from build123d import *

# Parameters (mm, degrees)
SKETCH1_W                = 59
SKETCH1_H                = 34
SKETCH1_W_2              = 55
SKETCH1_H_2              = 28
BOSS_EXTRUDE1_DEPTH      = 25
SKETCH1_2_W              = 55
SKETCH1_2_H              = 28
BOSS_EXTRUDE2_DEPTH      = 2
SKETCH2_W                = 2
SKETCH2_H                = 34
CUT_EXTRUDE1_DEPTH       = 25
SKETCH3_R                = 0.9
CUT_EXTRUDE2_DEPTH       = 25
CUT_EXTRUDE3_DEPTH       = 25
SKETCH5_W                = 2
SKETCH5_H                = 2
CUT_EXTRUDE4_DEPTH       = 51
SKETCH6_R                = 3.668845882
BOSS_EXTRUDE3_DEPTH      = 5.5
SKETCH4_3_R              = 2.4
CUT_EXTRUDE5_DEPTH       = 8
CUT_EXTRUDE5_TAPER       = -2
SKETCH7_W                = 24
SKETCH7_H                = 1.341552338
BOSS_EXTRUDE4_DEPTH      = 5.5
SKETCH8_R                = 1.5
CUT_EXTRUDE6_DEPTH       = 5.5
SKETCH9_W                = 10
SKETCH9_H                = 10
CUT_EXTRUDE7_DEPTH       = 2.5
SKETCH10_W               = 10
SKETCH10_H               = 10
CUT_EXTRUDE8_DEPTH       = 2.5
SKETCH11_R               = 1
CUT_EXTRUDE9_DEPTH       = 12.5
CUT_EXTRUDE9_DEPTH_BACK  = 2.5
SKETCH12_R               = 1
CUT_EXTRUDE10_DEPTH      = 12.5
CUT_EXTRUDE10_DEPTH_BACK = 2.5


with BuildPart() as part:
    # Sketch1 → Boss-Extrude1 (new body)
    with BuildSketch(Plane(origin=(0, 0, 0), x_dir=(1, 0, 0), z_dir=(0, 1, 0))):
        with Locations((29.5, 17)):
            Rectangle(SKETCH1_W, SKETCH1_H)
        with Locations((29.5, 17)):
            Rectangle(SKETCH1_W_2, SKETCH1_H_2, mode=Mode.SUBTRACT)
    extrude(amount=BOSS_EXTRUDE1_DEPTH)

    # Sketch1_2 → Boss-Extrude2 (add)
    with BuildSketch(Plane(origin=(0, 0, 0), x_dir=(1, 0, 0), z_dir=(0, 1, 0))):
        with Locations((29.5, 17)):
            Rectangle(SKETCH1_2_W, SKETCH1_2_H)
    extrude(amount=BOSS_EXTRUDE2_DEPTH)

    # Sketch2 → Cut-Extrude1 (cut)
    with BuildSketch(Plane(origin=(0, 25, 0), x_dir=(1, 0, 0), z_dir=(0, 1, 0))):
        with Locations((58, 17)):
            Rectangle(SKETCH2_W, SKETCH2_H)
    extrude(amount=-CUT_EXTRUDE1_DEPTH, mode=Mode.SUBTRACT)

    # Sketch3 → Cut-Extrude2 (cut)
    with BuildSketch(Plane(origin=(0, 2, 0), x_dir=(1, 0, 0), z_dir=(0, 1, 0))):
        with Locations((4, 9.5)):
            Circle(SKETCH3_R)
        with Locations((4, 24.5)):
            Circle(SKETCH3_R)
        with Locations((44.5, 9.5)):
            Circle(SKETCH3_R)
        with Locations((44.5, 24.5)):
            Circle(SKETCH3_R)
    extrude(amount=-CUT_EXTRUDE2_DEPTH, mode=Mode.SUBTRACT)

    # Sketch4 → Cut-Extrude3 (cut)
    with BuildSketch(Plane.ZY):
        with BuildLine():
            Line((-20.5, 3.8), (-13.5, 3.8))
            ThreePointArc((-13.5, 3.8), (-10.5, 6.8), (-13.5, 9.8))
            Line((-13.5, 9.8), (-20.5, 9.8))
            ThreePointArc((-20.5, 9.8), (-23.5, 6.8), (-20.5, 3.8))
        make_face()
        with BuildLine():
            Line((-24, 24.1), (-10, 24.1))
            ThreePointArc((-10, 24.1), (-9.4, 23.5), (-10, 22.9))
            Line((-10, 22.9), (-24, 22.9))
            ThreePointArc((-24, 22.9), (-24.6, 23.5), (-24, 24.1))
        make_face()
    extrude(amount=-CUT_EXTRUDE3_DEPTH, mode=Mode.SUBTRACT)

    # Sketch5 → Cut-Extrude4 (cut)
    with BuildSketch(Plane(origin=(57, 0, 0), x_dir=(0, 0, -1), z_dir=(1, 0, 0))):
        with Locations((2, 23)):
            Rectangle(SKETCH5_W, SKETCH5_H)
        with Locations((32, 23)):
            Rectangle(SKETCH5_W, SKETCH5_H)
    extrude(amount=-CUT_EXTRUDE4_DEPTH, mode=Mode.SUBTRACT)

    # Sketch6 → Boss-Extrude3 (add)
    with BuildSketch(Plane(origin=(2, 0, 0), x_dir=(0, 0, -1), z_dir=(1, 0, 0))):
        with Locations((17, 18)):
            Circle(SKETCH6_R)
    extrude(amount=BOSS_EXTRUDE3_DEPTH)

    # Sketch4_3 → Cut-Extrude5 (cut)
    with BuildSketch(Plane.ZY):
        with Locations((-17, 18)):
            Circle(SKETCH4_3_R)
        with BuildLine():
            ThreePointArc((-20.5, 9.8), (-23.5, 6.8), (-20.5, 3.8))
            Line((-20.5, 3.8), (-13.5, 3.8))
            ThreePointArc((-13.5, 3.8), (-10.5, 6.8), (-13.5, 9.8))
            Line((-13.5, 9.8), (-20.5, 9.8))
        make_face()
        with BuildLine():
            ThreePointArc((-24, 24.1), (-24.6, 23.5), (-24, 22.9))
            Line((-24, 22.9), (-10, 22.9))
            ThreePointArc((-10, 22.9), (-9.4, 23.5), (-10, 24.1))
            Line((-10, 24.1), (-24, 24.1))
        make_face()
    extrude(amount=-CUT_EXTRUDE5_DEPTH, taper=CUT_EXTRUDE5_TAPER, mode=Mode.SUBTRACT)

    # Sketch7 → Boss-Extrude4 (add)
    with BuildSketch(Plane(origin=(2, 0, 0), x_dir=(0, 0, -1), z_dir=(1, 0, 0))):
        with Locations((17, 21.329223831)):
            Rectangle(SKETCH7_W, SKETCH7_H)
    extrude(amount=BOSS_EXTRUDE4_DEPTH)

    # Sketch8 → Cut-Extrude6 (cut)
    with BuildSketch(Plane(origin=(0, 22, 0), x_dir=(1, 0, 0), z_dir=(0, 1, 0))):
        with Locations((5, 27)):
            Circle(SKETCH8_R)
        with Locations((5, 7)):
            Circle(SKETCH8_R)
    extrude(amount=-CUT_EXTRUDE6_DEPTH, mode=Mode.SUBTRACT)

    # Sketch9 → Cut-Extrude7 (cut)
    with BuildSketch(Plane(origin=(0, 0, -34), x_dir=(-1, 0, 0), z_dir=(0, 0, -1))):
        with Locations((-52, 13)):
            Rectangle(SKETCH9_W, SKETCH9_H)
    extrude(amount=-CUT_EXTRUDE7_DEPTH, mode=Mode.SUBTRACT)

    # Sketch10 → Cut-Extrude8 (cut)
    with BuildSketch(Plane.XY):
        with Locations((52, 13)):
            Rectangle(SKETCH10_W, SKETCH10_H)
    extrude(amount=-CUT_EXTRUDE8_DEPTH, mode=Mode.SUBTRACT)

    # Sketch11 → Cut-Extrude9 (cut, two sides)
    with BuildSketch(Plane(origin=(0, 18, 0), x_dir=(-1, 0, 0), z_dir=(0, -1, 0))) as cut_extrude9_sk:
        with Locations((-49, 1.3)):
            Circle(SKETCH11_R)
    extrude(amount=CUT_EXTRUDE9_DEPTH, mode=Mode.SUBTRACT)
    extrude(cut_extrude9_sk.sketch, amount=-CUT_EXTRUDE9_DEPTH_BACK, mode=Mode.SUBTRACT)

    # Sketch12 → Cut-Extrude10 (cut, two sides)
    with BuildSketch(Plane(origin=(0, 18, 0), x_dir=(-1, 0, 0), z_dir=(0, -1, 0))) as cut_extrude10_sk:
        with Locations((-48.8, 32.7)):
            Circle(SKETCH12_R)
    extrude(amount=CUT_EXTRUDE10_DEPTH, mode=Mode.SUBTRACT)
    extrude(cut_extrude10_sk.sketch, amount=-CUT_EXTRUDE10_DEPTH_BACK, mode=Mode.SUBTRACT)


solid = part.part
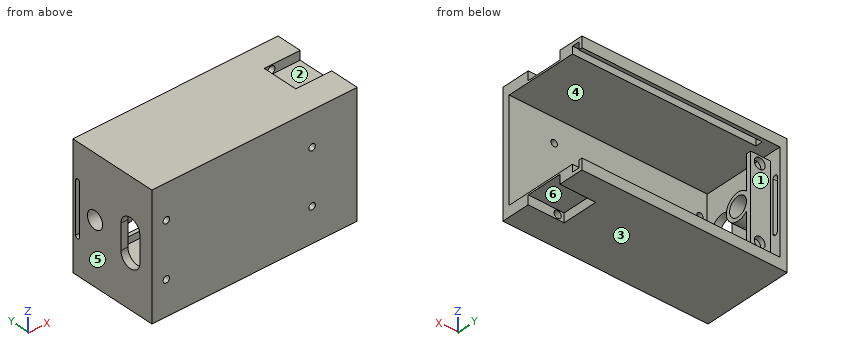
Work out the finished part from the listing and answer in its coordinate system (mm). Face numbers are marked on the shaded views. A direction names the side the tool comes from. Coordinates: 2 decimals unless noted, no trailing zeros. Write each loop counter-clockwise with the first axis right and the second up, starting at its lowest first coordinate (ties: lowest second). Pieces come first, ordered by that corner, then holes.
1. The part is cut by section D-D, the plane y = 11. Write down the section's boundary in (x, z), and give its area (3 significant figures).
Results list:
outline: (0, -34) - (47, -34) - (47, -31.5) - (57, -31.5) - (57, -31) - (2, -31) - (2, -3) - (57, -3) - (57, -2.5) - (47, -2.5) - (47, 0) - (0, 0) - close
area: 348 mm2
2. The part is cut by section A-A, the plane y = 6.8. Write down the section's boundary in (x, z).
Results list:
outline: (0, -34) - (57, -34) - (57, -31) - (2, -31) - (2, -23.57) - (0, -23.5) - close; (0, -10.5) - (2, -10.43) - (2, -3) - (57, -3) - (57, 0) - (0, 0) - close; hole circle Ø2 at (48.8, -32.7); hole circle Ø2 at (49, -1.3)
3. The part is cut by section C-C, the plane z = -4. Write down the section's boundary in (x, y), and give its area (3 significant figures).
Results list:
outline: (0, 0) - (57, 0) - (57, 2) - (2, 2) - (2, 25) - (0, 25) - close
area: 160 mm2
4. Consider line 1 along Z through (x, y) = (4, 1.55); line 2 along X through (y, z) = (1.1, -24.5); line 3 along Y through (x, z) = (49.5, -1.5). Determine where each line is inside the solid, lowest interval first.
Results list:
line 1: z = -34 to -25.4, -23.6 to -10.4, -8.6 to 0
line 2: x = 0 to 3.1, 4.9 to 43.6, 45.4 to 57
line 3: y = 0 to 5.5, 20.5 to 22, 24 to 25
5. For a pull along Y with two mould halves and no side action, classify the marked faces 1, 2 and 3 as +Y half, -Y half, draft (parallel to the pull), parting line (faces both ways), or undercut.
Results list:
face 1: +Y half
face 2: undercut
face 3: draft
6. Flat-ended cylindrical pins translate along their axes: pin 1 (4 mm diameter, centred on x = 45, z = -19, fed in from +Y); pin 2 (1.4 mm diameter, centred on x = 44.5, z = -9.5, fed in from -Y); pin 3 (1.2 mm diameter, centred on y = 10.5, z = -33, fed in from +X); pin 4 (1.1 mm diameter, centred on x = 4, z = -9.5, fed in from -Y). Find the tip coordinate at first contact, or state that the pin passes through.
Results list:
pin 1: stops at y = 2
pin 2: passes through
pin 3: stops at x = 47
pin 4: stops at y = 20.66
7. For the marked faces 4, 5 and 6, determine the directions among +Z, -Z, +X, -X, +Y, -Y from which every point of the face is accessible in a straight line to the end or side of a thin tool.
Results list:
face 4: +X, +Y
face 5: +Z, -Z, -X, +Y, -Y
face 6: -Z, +X
8. The part is cut by section B-B, the plane x = 44.5. Write down the section's boundary in (y, z), and give its area (3 significant figures).
Results list:
outline: (0, -34) - (25, -34) - (25, -31) - (24, -31) - (24, -33) - (22, -33) - (22, -31) - (2, -31) - (2, -25.4) - (0, -25.4) - close; (0, -23.6) - (2, -23.6) - (2, -10.4) - (0, -10.4) - close; (0, -8.6) - (2, -8.6) - (2, -3) - (22, -3) - (22, -1) - (24, -1) - (24, -3) - (25, -3) - (25, 0) - (0, 0) - close
area: 191 mm2
